Could you check a few things on this model? Use its own coordinates, in mm. Face numbers are marked on the shaded views. Give positions to 0.01 mm unless a question says otherwise; leave off trailing zeros. Write each loop counter-clockwise with the first axis right and the second up, starting at its lowest first coordinate (ties: lowest second). Pieces come first, ordered by that corner, then holes. Notation, with made-up numbers: (44.25, -28) - (62.25, -28) arc R21 cw to (62.25, 3) - close; hole circle Ø11 at (-7.5, 30.25). An arc over 180 degrees is marked (long way). Answer as CSV lines item,"result". Start each with the question number.
Q1. Imagine slicing it at A-A on x = 0. List the corners of the cut face in (y, z) for me, and give its area (3 significant figures).
Q2. We'd pull the mould along Z, two halves only. Please class the marked faces 1, 2 and 3: pulls with the +Z half, pulls with the -Z half, needs draft (parallel to the pull), parting line crosses it, or undercut.
Q3. Imagine slicing it at C-C on z = 335. List the corners of the cut face in (x, y) for me.
Q4. If I drill on line 1 along Z through (x, y) = (35, -57.5); line 2 along Z through (x, y) = (162, 99); line 3 along Y through (x, z) = (-25, 472), over which ranges is the centre line in solid material (lowest first)?
```python
from build123d import *

# Parameters (mm, degrees)
F2_R = 10
F3_R = 2


with BuildPart() as f1:
    # F0 (on Front) → F1 (revolve)
    with BuildSketch(Plane.XZ):
        Polygon((-150, 0), (0, 0), (0, 500), (-250, 500), (-250, 470), (-30, 470), (-30, 10), (-150, 10), align=None)
    revolve(axis=Axis((0, 0, 250), (0, 0, -1)))

    # F2
    f2_edges = [f1.edges().sort_by_distance(p)[0] for p in [
        (250, 0, 500),
        (250, 0, 470),
    ]]
    fillet(f2_edges, radius=F2_R)

    # F3
    f3_edges = [f1.edges().sort_by_distance(p)[0] for p in [
        (150, 0, 0),
        (150, 0, 10),
    ]]
    fillet(f3_edges, radius=F3_R)


solid = f1.part
```
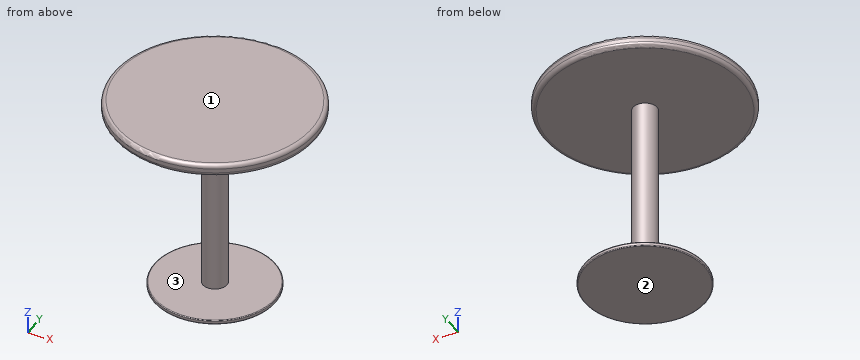
Conclusion:
1,outline,"(-250, 480) arc R10 ccw to (-240, 470) - (-30, 470) - (-30, 10) - (-148, 10) arc R2 ccw to (-150, 8) - (-150, 2) arc R2 ccw to (-148, 0) - (148, 0) arc R2 ccw to (150, 2) - (150, 8) arc R2 ccw to (148, 10) - (30, 10) - (30, 470) - (240, 470) arc R10 ccw to (250, 480) - (250, 490) arc R10 ccw to (240, 500) - (-240, 500) arc R10 ccw to (-250, 490) - close"
1,area,"45,500 mm^2"
2,face 1,"pulls with the +Z half"
2,face 2,"pulls with the -Z half"
2,face 3,"undercut"
3,outline,"circle Ø60 at (0, 0)"
4,line 1,"0 to 10, 470 to 500"
4,line 2,"470 to 500"
4,line 3,"-244.73 to 244.73"
